Geometry: final body of the model. Coordinates: model frame, mm. Face numbers are marked on the shaded views. Give positions to 0.01 mm unless a question says otherwise; leave off trailing zeros. Loops run counter-clockwise (first coordinate to the right, second up) from the corner with the lowest first, then second, coordinate; pieces in that order, holes last.
from build123d import *

# Parameters (mm, degrees)
F0_R     = 10.8782
F0_R_2   = 9.8782
F0_R_3   = 6.5
F0_R_4   = 5.4
F0_R_5   = 5
F1_DEPTH = 3
F2_DEPTH = 28.9814
F3_DEPTH = 4


with BuildPart() as f1:
    # F0 (on Top) → F1 (new body)
    with BuildSketch(Plane.XY):
        Circle(F0_R)
        Circle(F0_R_2, mode=Mode.SUBTRACT)
        Circle(F0_R_2)
        Circle(F0_R_3, mode=Mode.SUBTRACT)
        Circle(F0_R_3)
        Circle(F0_R_4, mode=Mode.SUBTRACT)
        Circle(F0_R_4)
        Circle(F0_R_5, mode=Mode.SUBTRACT)
        Circle(F0_R_5)
    extrude(amount=F1_DEPTH)

    # F0 (on Top) → F2 (join)
    with BuildSketch(Plane.XY):
        Circle(F0_R)
        Circle(F0_R_2, mode=Mode.SUBTRACT)
    extrude(amount=F2_DEPTH)

    # F0 (on Top) → F3 (join)
    with BuildSketch(Plane.XY):
        Circle(F0_R_5)
    extrude(amount=F3_DEPTH)


solid = f1.part
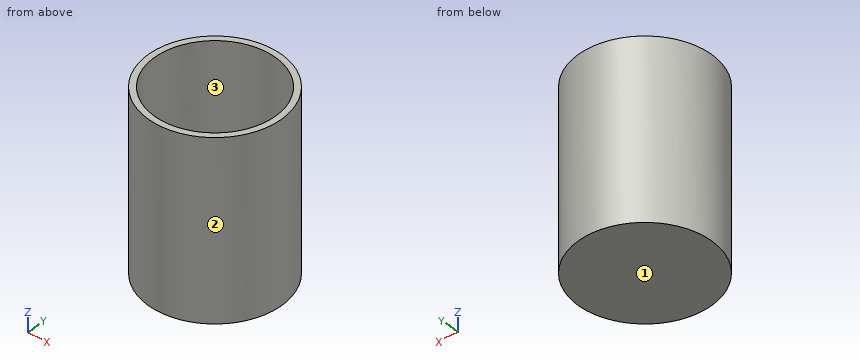
Item 1: Section query B-B on z = 8.75. Return loops of the section in (x, y), plus the area to 3 significant figures.
Values follow:
outline: circle Ø21.76 at (0, 0); hole circle Ø19.76 at (0, 0)
area: 65.2 mm2
Item 2: Section query D-D on x = 6.25. Return loops of the section in (y, z).
Values follow:
outline: (-8.9, 0) - (8.9, 0) - (8.9, 28.98) - (7.65, 28.98) - (7.65, 3) - (-7.65, 3) - (-7.65, 28.98) - (-8.9, 28.98) - close
Item 3: Section query A-A on x = 0. Return loops of the section in (y, z), plus the area to 3 significant figures.
Values follow:
outline: (-10.88, 0) - (10.88, 0) - (10.88, 28.98) - (9.88, 28.98) - (9.88, 3) - (5, 3) - (5, 4) - (-5, 4) - (-5, 3) - (-9.88, 3) - (-9.88, 28.98) - (-10.88, 28.98) - close
area: 127 mm2
Item 4: Pin query (flat end, axial travel): pin 1 (3 mm diameter, centred on x = -2.5, z = 13, fed in from +Y); pin 2 (3 mm diameter, centred on x = -2, y = 0, fed in from +Z); pin 3 (4 mm diameter, centred on x = 7, y = -3.5, fed in from +Z). Return the tip coordinate at first contact, or that it passes through.
Values follow:
pin 1: stops at y = 10.83
pin 2: stops at z = 4
pin 3: stops at z = 3
Item 5: Draft query along X for the marked faces 1, 2 and 3. Return one class per face: +X half, -X half, draft (parallel to the pull), parting line (faces both ways), or undercut.
Values follow:
face 1: draft
face 2: parting line
face 3: undercut
Item 6: Ray query, probe 1 along Y at (x, z) = (0, 13.5); probe 2 along Z at (x, y) = (3.75, 8.5). Return the intervals inside material, ascending.
Values follow:
probe 1: y = -10.88 to -9.88, 9.88 to 10.88
probe 2: z = 0 to 3
